from build123d import *

# Parameters (mm, degrees)
CROQUIS1_R              = 1.5
SALIENTE_EXTRUIR1_DEPTH = 2
CORTAR_EXTRUIR1_START   = -2
CORTAR_EXTRUIR1_DEPTH   = 2


with BuildPart() as part:
    # Croquis1 → Saliente-Extruir1 (new body)
    with BuildSketch(Plane.XY):
        with BuildLine():
            Line((-117.327111855, 45.850197678), (-96.327111855, 45.850197678))
            ThreePointArc((-96.327111855, 45.850197678), (-94.912898293, 46.435984115), (-94.327111855, 47.850197678))
            Line((-94.327111855, 47.850197678), (-94.327111855, 68.850197678))
            ThreePointArc((-94.327111855, 68.850197678), (-94.912898293, 70.26441124), (-96.327111855, 70.850197678))
            Line((-96.327111855, 70.850197678), (-117.327111855, 70.850197678))
            ThreePointArc((-117.327111855, 70.850197678), (-118.741325417, 70.26441124), (-119.327111855, 68.850197678))
            Line((-119.327111855, 68.850197678), (-119.327111855, 47.850197678))
            ThreePointArc((-119.327111855, 47.850197678), (-118.741325417, 46.435984115), (-117.327111855, 45.850197678))
        make_face()
        with Locations((-106.827111855, 58.350197678)):
            Circle(CROQUIS1_R, mode=Mode.SUBTRACT)
        with BuildLine():
            Line((-114.644626276, 68.350197678), (-114.644626276, 48.350197678))
            ThreePointArc((-114.644626276, 48.350197678), (-113.544626276, 47.250197678), (-112.444626276, 48.350197678))
            Line((-112.444626276, 48.350197678), (-112.444626276, 68.350197678))
            ThreePointArc((-112.444626276, 68.350197678), (-113.544626276, 69.450197678), (-114.644626276, 68.350197678))
        make_face(mode=Mode.SUBTRACT)
        with BuildLine():
            Line((-99.009597434, 48.350197678), (-99.009597434, 68.350197678))
            ThreePointArc((-99.009597434, 68.350197678), (-100.109597434, 69.450197678), (-101.209597434, 68.350197678))
            Line((-101.209597434, 68.350197678), (-101.209597434, 48.350197678))
            ThreePointArc((-101.209597434, 48.350197678), (-100.109597434, 47.250197678), (-99.009597434, 48.350197678))
        make_face(mode=Mode.SUBTRACT)
    extrude(amount=SALIENTE_EXTRUIR1_DEPTH)

    # Croquis2 → Cortar-Extruir1 (cut)
    with BuildSketch(Plane.XY.offset(2).offset(CORTAR_EXTRUIR1_START)):
        with BuildLine():
            Line((-96.327111855, 70.850197678), (-117.327111855, 70.850197678))
            ThreePointArc((-117.327111855, 70.850197678), (-118.741325417, 70.26441124), (-119.327111855, 68.850197678))
            Line((-119.327111855, 68.850197678), (-119.327111855, 47.850197678))
            ThreePointArc((-119.327111855, 47.850197678), (-118.741325417, 46.435984115), (-117.327111855, 45.850197678))
            Line((-117.327111855, 45.850197678), (-96.327111855, 45.850197678))
            ThreePointArc((-96.327111855, 45.850197678), (-94.912898293, 46.435984115), (-94.327111855, 47.850197678))
            Line((-94.327111855, 47.850197678), (-94.327111855, 68.850197678))
            ThreePointArc((-94.327111855, 68.850197678), (-94.912898293, 70.26441124), (-96.327111855, 70.850197678))
        make_face()
        with BuildLine():
            Line((-96.327111855, 70.500197678), (-117.327111855, 70.500197678))
            ThreePointArc((-117.327111855, 70.500197678), (-118.493838044, 70.016923867), (-118.977111855, 68.850197678))
            Line((-118.977111855, 68.850197678), (-118.977111855, 47.850197678))
            ThreePointArc((-118.977111855, 47.850197678), (-118.493838044, 46.683471489), (-117.327111855, 46.200197678))
            Line((-117.327111855, 46.200197678), (-96.327111855, 46.200197678))
            ThreePointArc((-96.327111855, 46.200197678), (-95.160385666, 46.683471489), (-94.677111855, 47.850197678))
            Line((-94.677111855, 47.850197678), (-94.677111855, 68.850197678))
            ThreePointArc((-94.677111855, 68.850197678), (-95.160385666, 70.016923867), (-96.327111855, 70.500197678))
        make_face(mode=Mode.SUBTRACT)
    extrude(amount=CORTAR_EXTRUIR1_DEPTH, mode=Mode.SUBTRACT)


solid = part.part
CAD build for the part. Positions are in the model's coordinates, mm. A direction names the side the tool comes from. Give positions to 0.01 mm unless a question says otherwise; leave off trailing zeros. Loops run counter-clockwise (first coordinate to the right, second up) from the corner with the lowest first, then second, coordinate; pieces in that order, holes last. Notation, with made-up numbers: M 60,60.25 L 107,60.25 A17 ccw 107,80.25 Z; hole C 30,-20 d6. An arc over 180 degrees is marked long. Write each question's results on one line, items separated by ' | '.
Q1. Flat gauge pin, fed straight in: P1, Ø2.5, axis at x = -106.83, y = 58.35, coming from the -Z side. Where does the tip first touch, or does it go through?
Geometry check:
P1: passes through
Q2. Band-saw the part on A-A on y = 61.5. Write the cut outline in (x, z), and give its area (3 significant figures).
Geometry check:
outline: M -118.98,0 L -114.64,0 L -114.64,2 L -118.98,2 Z; M -112.44,0 L -101.21,0 L -101.21,2 L -112.44,2 Z; M -99.01,0 L -94.68,0 L -94.68,2 L -99.01,2 Z | area: 39.8 mm²
Q3. Probe probe 1 along X at (y, z) = (48.5, 1.45); probe 2 along X at (y, z) = (47.5, 1.8); probe 3 along Y at (x, z) = (-106.25, 0.9). List the from-to ranges inside material, lowest first.
Geometry check:
probe 1: x = -118.98 to -114.64, -112.44 to -101.21, -99.01 to -94.68 | probe 2: x = -118.94 to -114.24, -112.85 to -100.81, -99.41 to -94.71 | probe 3: y = 46.2 to 56.97, 59.73 to 70.5
Q4. Band-saw the part on C-C on z = 0.8. Write the cut outline in (x, y).
Geometry check:
outline: M -118.98,47.85 A1.65 ccw -117.33,46.2 L -96.33,46.2 A1.65 ccw -94.68,47.85 L -94.68,68.85 A1.65 ccw -96.33,70.5 L -117.33,70.5 A1.65 ccw -118.98,68.85 Z; hole M -114.64,48.35 A1.1 ccw -112.44,48.35 L -112.44,68.35 A1.1 ccw -114.64,68.35 Z; hole C -106.83,58.35 d3; hole M -101.21,48.35 A1.1 ccw -99.01,48.35 L -99.01,68.35 A1.1 ccw -101.21,68.35 Z
Q5. Which spindle directions (+Z, -Z, +X, -X, +Y, -Y) get a long thin tool onto all of the face, cutting with end or side? Do faces 1 (the face through (-113.52, 69.45, 0.99)), 2 (the face through (-107, 46.2, 1)). Say none if no direction does.
Geometry check:
face 1: +Z, -Z | face 2: +Z, -Z, +X, -X, -Y
Q6. Mould opens along X. For faces 3 (the face through (-110, 59, 0)), 4 (the face through (-94.677, 58, 1)), 5 (the face through (-100.13, 47.25, 0.99)), 6 (the face through (-113.57, 47.25, 0.99)) say: pulls with the +X half, pulls with the -X half, needs draft (parallel to the pull), parting line crosses it, or undercut.
Geometry check:
face 3: needs draft | face 4: pulls with the +X half | face 5: undercut | face 6: undercut
Q7. Band-saw the part on B-B on x = -113.75. Write the cut outline in (y, z), and give its area (3 significant figures).
Geometry check:
outline: M 46.2,0 L 47.27,0 L 47.27,2 L 46.2,2 Z; M 69.43,0 L 70.5,0 L 70.5,2 L 69.43,2 Z | area: 4.28 mm²
Q8. Band-saw the part on D-D on y = 58. Write the cut outline in (x, z), and give its area (3 significant figures).
Geometry check:
outline: M -118.98,0 L -114.64,0 L -114.64,2 L -118.98,2 Z; M -112.44,0 L -108.29,0 L -108.29,2 L -112.44,2 Z; M -105.37,0 L -101.21,0 L -101.21,2 L -105.37,2 Z; M -99.01,0 L -94.68,0 L -94.68,2 L -99.01,2 Z | area: 34.0 mm²
